The model under review builds one solid part; all positions refer to its coordinate system, in mm. A direction names the side the tool comes from. Coordinates: 2 decimals unless noted, no trailing zeros. Loops run counter-clockwise (first coordinate to the right, second up) from the corner with the lowest first, then second, coordinate; pieces in that order, holes last. Notation, with made-up numbers: M 27.5,-8.75 L 35.5,-8.75 A28 ccw 35.5,18.25 Z; hole C -27.75,83.5 d10. An arc over 180 degrees is marked long. One line per item, written item: value.
```python
from build123d import *

# Parameters (mm, degrees)
SKETCH_W                = 90.24
SKETCH_H                = 65.24
SKETCH_R                = 1.778
PAD_DEPTH               = 5.08
POCKET_DEPTH            = 1.778
POCKET_MIRRORED_2_DEPTH = 1.778
SKETCH002_R             = 3.175
POCKET001_DEPTH         = 2.286
SKETCH003_W             = 1.905
SKETCH003_H             = 12.7
POCKET002_DEPTH         = 5.081
LINEARPATTERN_COUNT     = 8
LINEARPATTERN_PITCH     = 3.628571
FILLET_R                = 7.62
PAD001_DEPTH            = 0.635
SKETCH020_W             = 2.413
SKETCH020_H             = 32.512
PAD005_DEPTH            = 1.651


with BuildPart() as part:
    # Sketch → Pad (new body)
    with BuildSketch(Plane.XY):
        Rectangle(SKETCH_W, SKETCH_H)
        with Locations((37.5, 25)):
            Circle(SKETCH_R, mode=Mode.SUBTRACT)
        with Locations((-37.5, 25)):
            Circle(SKETCH_R, mode=Mode.SUBTRACT)
        with Locations((-37.5, -25)):
            Circle(SKETCH_R, mode=Mode.SUBTRACT)
        with Locations((37.5, -25)):
            Circle(SKETCH_R, mode=Mode.SUBTRACT)
    extrude(amount=PAD_DEPTH)

    # Sketch001 (on Face10 of Pad) → Pocket (cut)
    with BuildSketch(Plane.XY.offset(5.08)):
        with BuildLine():
            ThreePointArc((-37.5, 22.46), (-35.703949, 23.203949), (-34.96, 25))
            Line((-34.96, 25), (0, 25))
            Line((0, 0), (0, 25))
            Line((0, 0), (-37.5, 0))
            Line((-37.5, 0), (-37.5, 22.46))
        make_face()
    pocket = extrude(amount=-POCKET_DEPTH, mode=Mode.SUBTRACT)

    # Sketch001 Mirrored 2 → Pocket Mirrored 2 (cut)
    with BuildSketch(Plane(origin=(0, 0, 5.08), x_dir=(-1, 0, 0), z_dir=(0, 0, -1))):
        with BuildLine():
            ThreePointArc((-37.5, 22.46), (-35.703949, 23.203949), (-34.96, 25))
            Line((-34.96, 25), (0, 25))
            Line((0, 0), (0, 25))
            Line((0, 0), (-37.5, 0))
            Line((-37.5, 0), (-37.5, 22.46))
        make_face()
    pocket_mirrored_2 = extrude(amount=POCKET_MIRRORED_2_DEPTH, mode=Mode.SUBTRACT)

    # Mirrored001: Pocket, Pocket Mirrored 2 across Sketch001 H_Axis
    add(pocket.mirror(Plane(origin=(0, 0, 5.08), x_dir=(0, 0, 1), z_dir=(0, 1, 0))), mode=Mode.SUBTRACT)
    add(pocket_mirrored_2.mirror(Plane(origin=(0, 0, 5.08), x_dir=(0, 0, 1), z_dir=(0, 1, 0))), mode=Mode.SUBTRACT)

    # Sketch002 (on Face4 of MultiTransform) → Pocket001 (cut)
    with BuildSketch(Plane(origin=(0, 0, 0), x_dir=(1, 0, 0), z_dir=(0, 0, -1))):
        with Locations((37.5, 25)):
            Circle(SKETCH002_R)
        with Locations((-37.5, 25)):
            Circle(SKETCH002_R)
        with Locations((-37.5, -25)):
            Circle(SKETCH002_R)
        with Locations((37.5, -25)):
            Circle(SKETCH002_R)
    extrude(amount=-POCKET001_DEPTH, mode=Mode.SUBTRACT)

    # Sketch003 (on Face5 of Pocket001) → Pocket002 (cut, through all)
    with BuildSketch(Plane.XY.offset(5.08)):
        with Locations((25.5905, 21.844)):
            Rectangle(SKETCH003_W, SKETCH003_H)
    pocket002 = extrude(amount=-POCKET002_DEPTH, mode=Mode.SUBTRACT)

    # LinearPattern: Pocket002 ×8
    with Locations(*[(-i * LINEARPATTERN_PITCH, 0, 0) for i in range(1, LINEARPATTERN_COUNT)]):
        add(pocket002, mode=Mode.SUBTRACT)

    # Fillet
    fillet_edges = [part.edges().sort_by_distance(p)[0] for p in [
        (45.12, -32.62, 2.54),
        (-45.12, -32.62, 2.54),
        (-45.12, 32.62, 2.54),
        (45.12, 32.62, 2.54),
    ]]
    fillet(fillet_edges, radius=FILLET_R)

    # Sketch004 (on Face5 of Fillet) → Pad001 (join)
    with BuildSketch(Plane.XY.offset(5.08)):
        with BuildLine():
            Line((-37.5, -32.62), (37.5, -32.62))
            ThreePointArc((37.5, -32.62), (42.888154, -30.388154), (45.12, -25))
            Line((45.12, -25), (45.12, 25))
            ThreePointArc((45.12, 25), (42.888154, 30.388154), (37.5, 32.62))
            Line((37.5, 32.62), (-37.5, 32.62))
            ThreePointArc((-37.5, 32.62), (-42.888154, 30.388154), (-45.12, 25))
            Line((-45.12, 25), (-45.12, -25))
            ThreePointArc((-45.12, -25), (-42.888154, -30.388154), (-37.5, -32.62))
        make_face()
        with BuildLine():
            Line((-37.5, -31.35), (37.5, -31.35))
            ThreePointArc((37.5, -31.35), (41.990128, -29.490128), (43.85, -25))
            Line((43.85, -25), (43.85, 25))
            ThreePointArc((43.85, 25), (41.990128, 29.490128), (37.5, 31.35))
            Line((37.5, 31.35), (-37.5, 31.35))
            ThreePointArc((-37.5, 31.35), (-41.990128, 29.490128), (-43.85, 25))
            Line((-43.85, 25), (-43.85, -25))
            ThreePointArc((-43.85, -25), (-41.990128, -29.490128), (-37.5, -31.35))
        make_face(mode=Mode.SUBTRACT)
    extrude(amount=PAD001_DEPTH)

    # Sketch020 (on Face58 of Pad001) → Pad005 (join)
    with BuildSketch(Plane.XY.offset(5.08)):
        with Locations((43.9135, 0)):
            Rectangle(SKETCH020_W, SKETCH020_H)
    extrude(amount=PAD005_DEPTH)


with BuildPart() as part_1:
    # Body placement: moved
    add(part.part.moved(Location((0, 0, -5.207))))


solid = part_1.part
```
(1) Add section C-C on y = 29.5. State the section outline as (x, z) points.
Checks:
outline: M -43.65,-5.21 L 43.65,-5.21 L 43.65,0.51 L 41.98,0.51 L 41.98,-0.13 L -41.98,-0.13 L -41.98,0.51 L -43.65,0.51 Z
(2) Insertion check: pin 1 Ø7.5 at (x, y) = (-37.5, 25) entering from +Z; pin 2 Ø3 at (x, y) = (37.5, -25) entering from +Z; pin 3 Ø15 at (x, y) = (-16, 8) entering from +Z (3 decimals). Each pin has a flat end and moves straight along its axis. Give the tip position at first contact, or say it passes through.
Checks:
pin 1: z = -0.13
pin 2: through
pin 3: z = -1.905
(3) Add section B-B on x = -19. State the section outline as (y, z) points (3 decimals), then the cut area to 3 significant figures.
Checks:
outline: M -32.62,-5.207 L 32.62,-5.207 L 32.62,0.508 L 31.35,0.508 L 31.35,-0.127 L 25,-0.127 L 25,-1.905 L -25,-1.905 L -25,-0.127 L -31.35,-0.127 L -31.35,0.508 L -32.62,0.508 Z
area: 244 mm^2
(4) Draft analysis for pull direction Y (two halves, no side actions). For faces 1 (the face through (45.12, 0, -2)), 2 (the face through (11, 28.194, -3)), state which applies: pulls with the +Y half, pulls with the -Y half, needs draft (parallel to the pull), parting line crosses it, or undercut.
Checks:
face 1: needs draft
face 2: undercut
(5) Add section A-A on y = 10. State the section outline as (x, z) points (3 decimals), then the cut area to 3 significant figures.
Checks:
outline: M -45.12,-5.207 L 45.12,-5.207 L 45.12,1.524 L 42.707,1.524 L 42.707,-0.127 L 37.5,-0.127 L 37.5,-1.905 L -37.5,-1.905 L -37.5,-0.127 L -43.85,-0.127 L -43.85,0.508 L -45.12,0.508 Z
area: 330 mm^2
(6) To check wall thickness, follow L1, parallel to Y at x = -37.5, z = -4 (3 decimals); L2, parallel to Y at x = -37.5, z = -2.35; L3, parallel to X at y = -25, z = -4.05 (3 decimals). State the ranges of each line that lie inside material, in increasing order. Write a range as [from, to].
Checks:
L1: [-32.62, -28.175], [-21.825, 21.825], [28.175, 32.62]
L2: [-32.62, -26.78], [-23.22, 23.22], [26.78, 32.62]
L3: [-45.12, -40.675], [-34.325, 34.325], [40.675, 45.12]
(7) Tool access review of faces 3 (the face through (12.029, 22, -3)), 4 (the face through (35.724, 23.184, -1.004)), 5 (the face through (-36.1, -23.6, -2.921)): name each direction out of +Z, -Z, +X, -X, +Y, -Y from which nothing blocks a thin tool from reaching the whole face with its end or side.
Checks:
face 3: +Z, -Z
face 4: +Z
face 5: -Z
